Input: part model. Units: mm. Frame: model coordinates. A direction names the side the tool comes from. Coordinates: 2 decimals unless noted, no trailing zeros. Order: outer loops, then holes, each group sorted by start corner. A loop starts at its lowest first (then second) coordinate and runs counter-clockwise, first axis right, second up. Notation, with made-up numbers: (11.25, -14) - (45.25, -14) arc R5 ccw to (45.25, -9) - close; hole circle Ø5 at (33.25, 53). An arc over 180 degrees is marked (long way). Answer as CSV lines item,"result". Start each with the question number.
Item 1: Draft query along Z for faces 3 (the flat face through (-3, 4, -152)), 4 (the flat face through (178, 3, 2)), 5 (the flat face through (-3, 0, -2)). Return one class per face: +Z half, -Z half, draft (parallel to the pull), parting line (faces both ways), or undercut.
Item 2: First-contact query: pin 1 (4 mm diameter, centred on x = -57.5, z = 48, fed in from +Y); pin 2 (2 mm diameter, centred on x = 160, y = 4, fed in from +Z); pin 3 (5 mm diameter, centred on x = -178, z = 48.5, fed in from +Y); pin 4 (0.5 mm diameter, centred on y = 3, z = 128, fed in from +X). Flat tips, straight axial feed; report the tip coordinate or a pass-through.
Item 3: Section B-B (z = 55.5). Output: boundary loops of the cut face in (x, y), and give its area (4 significant figures).
Item 4: Section A-A (x = -151). Output: boundary loops of the cut face in (y, z), and give its area (3 significant figures).
Item 5: Access query for faces 1 (the flat face through (113, 3, 2)), 2 (the flat face through (192.5, 4, 2)). Directions: +Z, -Z, +X, -X, +Y, -Y. A direction counts if a zero-diameter tool reaches every point of the face in a straight line with its end or side. Return the directions, or none.
Item 6: Material intervals for line 1 along Z through (x, y) = (-186.25, 4); line 2 along X through (y, z) = (0.75, -47.5); line 3 along Y through (x, z) = (-96, -149), sorted ascending.
from build123d import *

# Parameters (mm, degrees)
SKETCH1_W           = 385
SKETCH1_H           = 304
EXTRUDE1_DEPTH      = 8
SKETCH2_R           = 1.65
CUT_EXTRUDE1_DEPTH  = 9.5
SKETCH3_R           = 1.65
CUT_EXTRUDE2_DEPTH  = 10
SKETCH4_W           = 365
SKETCH4_H           = 284
CUT_EXTRUDE3_DEPTH  = 5
SKETCH5_W           = 10
SKETCH5_H           = 284
BOSS_EXTRUDE1_DEPTH = 5
SKETCH6_W           = 10
SKETCH6_H           = 284
BOSS_EXTRUDE2_DEPTH = 5
SKETCH7_R           = 1.65
CUT_EXTRUDE4_DEPTH  = 10
MIRROR3_OUTLINE_R   = 1.65
MIRROR3_DEPTH       = 8
MIRROR3_START       = 3
MIRROR3_2_OUTLINE_W = 10
MIRROR3_2_OUTLINE_H = 284
MIRROR3_2_OUTLINE_R = 1.65
MIRROR3_2_DEPTH     = 5
FILLET1_R           = 5


# Read off the part's stored shape, not the designer's step: Mirror3
with BuildPart() as part:
    # Sketch1 → Extrude1 (new body)
    with BuildSketch(Plane(origin=(0, 0, 0), x_dir=(1, 0, 0), z_dir=(0, 1, 0))):
        Rectangle(SKETCH1_W, SKETCH1_H)
    extrude(amount=EXTRUDE1_DEPTH)

    # Sketch2 → Cut-Extrude1 (cut)
    with BuildSketch(Plane.XY.offset(152)):
        with Locations((-160, 4)):
            Circle(SKETCH2_R)
        with Locations((-96, 4)):
            Circle(SKETCH2_R)
        with Locations((-32, 4)):
            Circle(SKETCH2_R)
        with Locations((32, 4)):
            Circle(SKETCH2_R)
        with Locations((96, 4)):
            Circle(SKETCH2_R)
        with Locations((160, 4)):
            Circle(SKETCH2_R)
    cut_extrude1 = extrude(amount=-CUT_EXTRUDE1_DEPTH, mode=Mode.SUBTRACT)

    # Mirror1: Cut-Extrude1 across plane
    add(cut_extrude1.mirror(Plane.XY), mode=Mode.SUBTRACT)

    # Sketch3 → Cut-Extrude2 (cut)
    with BuildSketch(Plane.ZY.offset(192.5)):
        with Locations((-128, 4)):
            Circle(SKETCH3_R)
        with Locations((-64, 4)):
            Circle(SKETCH3_R)
        with Locations((0, 4)):
            Circle(SKETCH3_R)
        with Locations((64, 4)):
            Circle(SKETCH3_R)
        with Locations((128, 4)):
            Circle(SKETCH3_R)
    cut_extrude2 = extrude(amount=-CUT_EXTRUDE2_DEPTH, mode=Mode.SUBTRACT)

    # Mirror2: Cut-Extrude2 across plane
    add(cut_extrude2.mirror(Plane(origin=(0, 0, 0), x_dir=(0, 0, 1), z_dir=(1, 0, 0))), mode=Mode.SUBTRACT)

    # Sketch4 → Cut-Extrude3 (cut)
    with BuildSketch(Plane(origin=(0, 8, 0), x_dir=(-1, 0, 0), z_dir=(0, 1, 0))):
        Rectangle(SKETCH4_W, SKETCH4_H)
    extrude(amount=-CUT_EXTRUDE3_DEPTH, mode=Mode.SUBTRACT)

    # Sketch5 → Boss-Extrude1 (add)
    with BuildSketch(Plane(origin=(0, 3, 0), x_dir=(1, 0, 0), z_dir=(0, 1, 0))):
        with Locations((-167.5, 0)):
            Rectangle(SKETCH5_W, SKETCH5_H)
        with Locations((167.5, 0)):
            Rectangle(SKETCH5_W, SKETCH5_H)
    boss_extrude1 = extrude(amount=BOSS_EXTRUDE1_DEPTH)

    # Sketch6 → Boss-Extrude2 (add)
    with BuildSketch(Plane(origin=(0, 3, 0), x_dir=(1, 0, 0), z_dir=(0, 1, 0))):
        Rectangle(SKETCH6_W, SKETCH6_H)
    extrude(amount=BOSS_EXTRUDE2_DEPTH)

    # Sketch7 → Cut-Extrude4 (cut)
    with BuildSketch(Plane(origin=(0, 8, 0), x_dir=(1, 0, 0), z_dir=(0, 1, 0))):
        with Locations(Location((-167.5, -112, 0), (0, 0, 270))):
            Circle(SKETCH7_R)
        with Locations(Location((-167.5, -80, 0), (0, 0, 270))):
            Circle(SKETCH7_R)
        with Locations(Location((-167.5, -48, 0), (0, 0, 270))):
            Circle(SKETCH7_R)
        with Locations(Location((-167.5, -16, 0), (0, 0, 270))):
            Circle(SKETCH7_R)
        with Locations(Location((-167.5, 16, 0), (0, 0, 270))):
            Circle(SKETCH7_R)
        with Locations(Location((-167.5, 48, 0), (0, 0, 270))):
            Circle(SKETCH7_R)
        with Locations(Location((-167.5, 80, 0), (0, 0, 270))):
            Circle(SKETCH7_R)
        with Locations(Location((-167.5, 112, 0), (0, 0, 270))):
            Circle(SKETCH7_R)
        with Locations(Location((167.5, 112, 0), (0, 0, 270))):
            Circle(SKETCH7_R)
        with Locations(Location((167.5, 80, 0), (0, 0, 270))):
            Circle(SKETCH7_R)
        with Locations(Location((167.5, 48, 0), (0, 0, 270))):
            Circle(SKETCH7_R)
        with Locations(Location((167.5, 16, 0), (0, 0, 270))):
            Circle(SKETCH7_R)
        with Locations(Location((167.5, -16, 0), (0, 0, 270))):
            Circle(SKETCH7_R)
        with Locations(Location((167.5, -48, 0), (0, 0, 270))):
            Circle(SKETCH7_R)
        with Locations(Location((167.5, -80, 0), (0, 0, 270))):
            Circle(SKETCH7_R)
        with Locations(Location((167.5, -112, 0), (0, 0, 270))):
            Circle(SKETCH7_R)
        with Locations(Location((-167.5, 144, 0), (0, 0, 270))):
            Circle(SKETCH7_R)
        with Locations(Location((-167.5, -144, 0), (0, 0, 270))):
            Circle(SKETCH7_R)
        with Locations(Location((167.5, -144, 0), (0, 0, 270))):
            Circle(SKETCH7_R)
        with Locations(Location((167.5, 144, 0), (0, 0, 270))):
            Circle(SKETCH7_R)
    cut_extrude4 = extrude(amount=-CUT_EXTRUDE4_DEPTH, mode=Mode.SUBTRACT)

    # Mirror3 outline → Mirror3 (cut)
    with BuildSketch(Plane(origin=(0, 0, 0), x_dir=(1, 0, 0), z_dir=(0, 1, 0))):
        with Locations((-57.5, -112)):
            Circle(MIRROR3_OUTLINE_R)
        with Locations((-57.5, -80)):
            Circle(MIRROR3_OUTLINE_R)
        with Locations((-57.5, -48)):
            Circle(MIRROR3_OUTLINE_R)
        with Locations((-57.5, -16)):
            Circle(MIRROR3_OUTLINE_R)
        with Locations((-57.5, 16)):
            Circle(MIRROR3_OUTLINE_R)
        with Locations((-57.5, 48)):
            Circle(MIRROR3_OUTLINE_R)
        with Locations((-57.5, 80)):
            Circle(MIRROR3_OUTLINE_R)
        with Locations((-57.5, 112)):
            Circle(MIRROR3_OUTLINE_R)
        with Locations((-57.5, 144)):
            Circle(MIRROR3_OUTLINE_R)
        with Locations((-57.5, -144)):
            Circle(MIRROR3_OUTLINE_R)
    mirror3 = extrude(amount=MIRROR3_DEPTH, mode=Mode.SUBTRACT)

    # Mirror3 2 outline → Mirror3 2 (add)
    with BuildSketch(Plane(origin=(0, 0, 0), x_dir=(1, 0, 0), z_dir=(0, 1, 0)).offset(MIRROR3_START)):
        with Locations((-57.5, 0)):
            Rectangle(MIRROR3_2_OUTLINE_W, MIRROR3_2_OUTLINE_H)
        with Locations((-57.5, -112)):
            Circle(MIRROR3_2_OUTLINE_R, mode=Mode.SUBTRACT)
        with Locations((-57.5, -80)):
            Circle(MIRROR3_2_OUTLINE_R, mode=Mode.SUBTRACT)
        with Locations((-57.5, -48)):
            Circle(MIRROR3_2_OUTLINE_R, mode=Mode.SUBTRACT)
        with Locations((-57.5, -16)):
            Circle(MIRROR3_2_OUTLINE_R, mode=Mode.SUBTRACT)
        with Locations((-57.5, 16)):
            Circle(MIRROR3_2_OUTLINE_R, mode=Mode.SUBTRACT)
        with Locations((-57.5, 48)):
            Circle(MIRROR3_2_OUTLINE_R, mode=Mode.SUBTRACT)
        with Locations((-57.5, 80)):
            Circle(MIRROR3_2_OUTLINE_R, mode=Mode.SUBTRACT)
        with Locations((-57.5, 112)):
            Circle(MIRROR3_2_OUTLINE_R, mode=Mode.SUBTRACT)
    mirror3_2 = extrude(amount=MIRROR3_2_DEPTH)

    # Mirror4: Boss-Extrude1, Cut-Extrude4, Mirror3, Mirror3 2 across plane
    add(boss_extrude1.mirror(Plane(origin=(0, 0, 0), x_dir=(0, 0, 1), z_dir=(1, 0, 0))))
    add(cut_extrude4.mirror(Plane(origin=(0, 0, 0), x_dir=(0, 0, 1), z_dir=(1, 0, 0))), mode=Mode.SUBTRACT)
    add(mirror3.mirror(Plane(origin=(0, 0, 0), x_dir=(0, 0, 1), z_dir=(1, 0, 0))), mode=Mode.SUBTRACT)
    add(mirror3_2.mirror(Plane(origin=(0, 0, 0), x_dir=(0, 0, 1), z_dir=(1, 0, 0))))

    # Fillet1
    fillet1_edges = [part.edges().sort_by_distance(p)[0] for p in [
        (182.5, 5.5, -142),
        (182.5, 5.5, 142),
        (-182.5, 5.5, 142),
        (-182.5, 5.5, -142),
        (-172.5, 5.5, -142),
        (-172.5, 5.5, 142),
        (-162.5, 5.5, 142),
        (-162.5, 5.5, -142),
        (172.5, 5.5, -142),
        (162.5, 5.5, -142),
        (162.5, 5.5, 142),
        (172.5, 5.5, 142),
        (-5, 5.5, -142),
        (-5, 5.5, 142),
        (5, 5.5, 142),
        (5, 5.5, -142),
        (-62.5, 5.5, 142),
        (-62.5, 5.5, -142),
        (-52.5, 5.5, -142),
        (-52.5, 5.5, 142),
        (52.5, 5.5, -142),
        (52.5, 5.5, 142),
        (62.5, 5.5, 142),
        (62.5, 5.5, -142),
    ]]
    fillet(fillet1_edges, radius=FILLET1_R - 0.0001)  # a hair under: the kernel refuses the full size


solid = part.part
Determined:
1,face 3,"-Z half"
1,face 4,"undercut"
1,face 5,"draft"
2,pin 1,"stops at y = 8"
2,pin 2,"stops at z = 142.5"
2,pin 3,"stops at y = 3"
2,pin 4,"stops at x = 182.5"
3,outline,"(-192.5, 0) - (192.5, 0) - (192.5, 8) - (182.5, 8) - (182.5, 3) - (172.5, 3) - (172.5, 8) - (162.5, 8) - (162.5, 3) - (62.5, 3) - (62.5, 8) - (52.5, 8) - (52.5, 3) - (5, 3) - (5, 8) - (-5, 8) - (-5, 3) - (-52.5, 3) - (-52.5, 8) - (-62.5, 8) - (-62.5, 3) - (-162.5, 3) - (-162.5, 8) - (-172.5, 8) - (-172.5, 3) - (-182.5, 3) - (-182.5, 8) - (-192.5, 8) - close"
3,area,"1,505 mm^2"
4,outline,"(0, -152) - (8, -152) - (8, -142) - (3, -142) - (3, 142) - (8, 142) - (8, 152) - (0, 152) - close"
4,area,"1,010 mm^2"
5,face 1,"+Y"
5,face 2,"+Z, -Z, +X, +Y, -Y"
6,line 1,"z = -152 to -129.65, -126.35 to -65.65, -62.35 to -1.65, 1.65 to 62.35, 65.65 to 126.35, 129.65 to 152"
6,line 2,"x = -192.5 to -169.07, -165.93 to -59.07, -55.93 to 55.93, 59.07 to 165.93, 169.07 to 192.5"
6,line 3,"y = 0 to 2.35, 5.65 to 8"
